```python
from build123d import *

# Parameters (mm, degrees)
F1_DEPTH   = 90
F4_D       = 9
F4_ON_F2_D = 9


with BuildPart() as f1:
    # F0 (on Right) → F1 (new body)
    with BuildSketch(Plane.YZ):
        Polygon((-51, 0), (0, 0), (0, 51), (-9, 51), (-9, 31), (-19.6464466094, 20.3535533906), (-16.1109127035, 16.8180194847), (-5, 27.9289321881), (-5, 5), (-27.9289321881, 5), (-16.8180194847, 16.1109127035), (-20.3535533906, 19.6464466094), (-31, 9), (-51, 9), align=None)
    extrude(amount=F1_DEPTH)

    # F4 (through all)
    with Locations(Plane(origin=(0, 0, 0), x_dir=(1, 0, 0), z_dir=(0, 0, -1))):
        with Locations((70, 41), (20, 41)):
            Hole(F4_D / 2)

    # F4 on F2 (through all)
    with Locations(Plane(origin=(0, 0, 0), x_dir=(-1, 0, 0), z_dir=(0, 1, 0))):
        with Locations((-20, 41), (-70, 41)):
            Hole(F4_ON_F2_D / 2)


solid = f1.part
```
Can you work these out from the model? Positions are in its coordinate system, mm. A direction names the side the tool comes from. Give positions to 0.01 mm unless a question says otherwise; leave off trailing zeros. Write each loop counter-clockwise with the first axis right and the second up, starting at its lowest first coordinate (ties: lowest second). Pieces come first, ordered by that corner, then holes. Notation, with made-up numbers: (79.25, 12) -> (123.25, 12) arc R7 ccw to (123.25, 19) -> close; hole circle Ø5 at (29.5, 51.5). An arc over 180 degrees is marked (long way). Write item = value, one per line.
(1) I'm going to push flat-ended pins straight in: P1, Ø14.5, axis at x = 70, z = 41, coming from the -Y side; P2, Ø12, axis at x = 55.5, y = -30.5, coming from the -Z side; P3, Ø2, axis at x = 74.5, y = -24, coming from the +Z side; P4, Ø14.5, axis at x = 70, y = -41, coming from the +Z side. Where does each tip first touch, or does it pass through?
Worked out:
P1 = -9
P2 = 0
P3 = 17
P4 = 9
(2) Suppose I cut it at B-B on y = -41. Write out the boundary of the cut face in (x, z), then the cut area to 3 significant figures.
Worked out:
outline = (0, 0) -> (15.5, 0) -> (15.5, 9) -> (0, 9) -> close; (24.5, 0) -> (65.5, 0) -> (65.5, 9) -> (24.5, 9) -> close; (74.5, 0) -> (90, 0) -> (90, 9) -> (74.5, 9) -> close
area = 648 mm^2
(3) Suppose I cut it at C-C on z = 6. Write out the boundary of the cut face in (x, y), then the cut area to 3 significant figures.
Worked out:
outline = (0, -51) -> (90, -51) -> (90, -26.93) -> (0, -26.93) -> close; (0, -5) -> (90, -5) -> (90, 0) -> (0, 0) -> close; hole circle Ø9 at (20, -41); hole circle Ø9 at (70, -41)
area = 2,490 mm^2
(4) I need wall thicknesses on probe 1 along X at (y, z) = (-41, 4); probe 2 along Y at (x, z) = (20, 2.25); probe 3 along Y at (x, z) = (41.5, 17). Which ranges of each line are inside material? Lowest first, please. Write a range as from..to.
Worked out:
probe_1 = 0..15.5, 24.5..65.5, 74.5..90
probe_2 = -51..-45.5, -36.5..0
probe_3 = -23..-17.71, -16.29..-15.93, -5..0
(5) Suppose I cut it at D-D on x = 52.5. Write out the boundary of the cut face in (y, z), then the cut area to 3 significant figures.
Worked out:
outline = (-51, 0) -> (0, 0) -> (0, 51) -> (-9, 51) -> (-9, 31) -> (-19.65, 20.35) -> (-16.11, 16.82) -> (-5, 27.93) -> (-5, 5) -> (-27.93, 5) -> (-16.82, 16.11) -> (-20.35, 19.65) -> (-31, 9) -> (-51, 9) -> close
area = 811 mm^2
(6) For faces 1 (the face through (44.37, -22.45, 10.48)), 2 (the face through (44, -9, 41)), 3 (the face through (44, -26, 0)), which set-ups out of +Z, -Z, +X, -X, +Y, -Y let a thin tool reach every point of the face, with its end or its side?
Worked out:
face_1 = +X, -X
face_2 = +Z, +X, -X, -Y
face_3 = -Z, +X, -X, +Y, -Y
(7) Thinking about a two-plate mould opening in X: for faces 4 (the face through (44, -16, 5)), 5 (the face through (67.92, -37.01, 4.56)), 6 (the face through (0, -20, 14)), which applies, released by +X, released by -X, zero draft, split by the parting line, or undercut?
Worked out:
face_4 = zero draft
face_5 = undercut
face_6 = released by -X
(8) Suppose I cut it at A-A on x = 20. Write out the boundary of the cut face in (y, z).
Worked out:
outline = (-51, 0) -> (-45.5, 0) -> (-45.5, 9) -> (-51, 9) -> close; (-36.5, 0) -> (0, 0) -> (0, 36.5) -> (-9, 36.5) -> (-9, 31) -> (-19.65, 20.35) -> (-16.11, 16.82) -> (-5, 27.93) -> (-5, 5) -> (-27.93, 5) -> (-16.82, 16.11) -> (-20.35, 19.65) -> (-31, 9) -> (-36.5, 9) -> close; (-9, 45.5) -> (0, 45.5) -> (0, 51) -> (-9, 51) -> close
